Model file for the job. Use its own axes, mm. Face numbers are marked on the shaded views. A direction names the side the tool comes from. Give positions to 0.01 mm unless a question says otherwise; leave off trailing zeros. Loops run counter-clockwise (first coordinate to the right, second up) from the corner with the lowest first, then second, coordinate; pieces in that order, holes last. Notation, with made-up numbers: M 14,18 L 65,18 A24 ccw 65,51 Z; hole C 27.25,85 d7. An arc over 180 degrees is marked long. Use CSV: the item, a comma, the result in double quotes. Start each with the question number.
(1) Two-plate mould, pull along X, no slides. Class the marked faces 1, 2 and 3: pulls with the +X half, pulls with the -X half, needs draft (parallel to the pull), parting line crosses it, or undercut.
(2) Flat gauge pins, fed straight in: P1, Ø1.2, axis at x = -3, y = 15.5, coming from the -Z side; P2, Ø2, axis at x = 1, y = 7.5, coming from the +Z side; P3, Ø3, axis at x = -3, y = 2.5, coming from the -Z side; P4, Ø3, axis at x = 1.5, z = 0.5, coming from the -Y side. Where does each tip first touch, or does it go through?
(3) Wall check: line 1 along X through (y, z) = (14.75, 3.25); line 2 along Z through (x, y) = (1.25, 10.75); line 3 along Y through (x, z) = (0.25, 1.5). Give the ranges that are in metal, low to high. Write a range as from..to.
(4) Slice it at C-C on y = 7. List the corners of the cut face in (x, z).
(5) Tool access for the marked faces 4 and 5: list every direction of +Z, -Z, +X, -X, +Y, -Y with a clear straight run to the whole face (end or side of a thin tool).
(6) Slice it at D-D on y = 14. List the corners of the cut face in (x, z), and give its area (3 significant figures).
(7) Slice it at A-A on x = 0. List the corners of the cut face in (y, z), and give its area (4 significant figures).
(8) Slice it at B-B on z = 0. List the corners of the cut face in (x, y).
```python
from build123d import *

# Parameters (mm, degrees)
SKETCH1_R           = 3
BOSS_EXTRUDE1_DEPTH = 13
CUT_EXTRUDE1_DEPTH  = 1.5
FILLET1_R           = 1
FILLET2_R           = 1
FILLET3_R           = 1
FILLET4_R           = 1


with BuildPart() as part:
    # Sketch1 → Boss-Extrude1 (new body)
    with BuildSketch(Plane(origin=(0, 0, 0), x_dir=(1, 0, 0), z_dir=(0, 1, 0))):
        with Locations(Location((0, 0, 0), (0, 0, 90))):
            Circle(SKETCH1_R)
    extrude(amount=BOSS_EXTRUDE1_DEPTH)

    # Sketch3 → Revolve2 (revolve)
    with BuildSketch(Plane.XY, mode=Mode.PRIVATE) as revolve2_sk:
        Polygon((0, 13), (0, 16), (-5.5, 16), (-3, 13), align=None)
    revolve(revolve2_sk.sketch.rotate(Axis((0, 13, 0), (0, 1, 0)), 270), axis=Axis((0, 13, 0), (0, 1, 0)))

    # Sketch4 → Cut-Extrude1 (cut)
    with BuildSketch(Plane(origin=(0, 16, 0), x_dir=(1, 0, 0), z_dir=(0, 1, 0))):
        Polygon((-0.819580165, 0.819580165), (-3.693115778, 0.819580165), (-3.693115778, -0.819580165), (-0.819580165, -0.819580165), (-0.819580165, -3.693115778), (0.819580165, -3.693115778), (0.819580165, -0.819580165), (3.693115778, -0.819580165), (3.693115778, 0.819580165), (0.819580165, 0.819580165), (0.819580165, 3.693115778), (-0.819580165, 3.693115778), align=None)
    extrude(amount=-CUT_EXTRUDE1_DEPTH, mode=Mode.SUBTRACT)

    # Fillet1
    fillet1_edges = [part.edges().sort_by_distance(p)[0] for p in [
        (0, 14.5, -3.693115778),
    ]]
    fillet(fillet1_edges, radius=FILLET1_R)

    # Fillet2
    fillet2_edges = [part.edges().sort_by_distance(p)[0] for p in [
        (3.693115778, 14.5, 0),
    ]]
    fillet(fillet2_edges, radius=FILLET2_R)

    # Fillet3
    fillet3_edges = [part.edges().sort_by_distance(p)[0] for p in [
        (0, 14.5, 3.693115778),
    ]]
    fillet(fillet3_edges, radius=FILLET3_R)

    # Fillet4
    fillet4_edges = [part.edges().sort_by_distance(p)[0] for p in [
        (-3.693115778, 14.5, 0),
    ]]
    fillet(fillet4_edges, radius=FILLET4_R)


solid = part.part
```
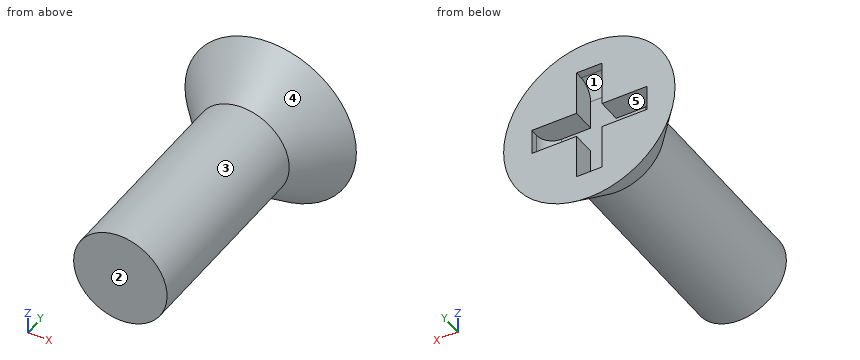
Reply:
1,face 1,"undercut"
1,face 2,"needs draft"
1,face 3,"parting line crosses it"
2,P1,"stops at z = -4.81"
2,P2,"stops at z = 3"
2,P3,"stops at z = -2.6"
2,P4,"stops at y = 0"
3,line 1,"x = -3.05..-0.82, 0.82..3.05"
3,line 2,"z = -2.73..2.73"
3,line 3,"y = 0..14.5"
4,outline,"C 0,0 d6"
5,face 4,"-Y"
5,face 5,"+Y"
6,outline,"C 0,0 d7.67"
6,area,"46.2 mm^2"
7,outline,"M 0,-3 L 13,-3 L 16,-5.5 L 16,-3.69 L 15.5,-3.69 A1 cw 14.5,-2.69 L 14.5,2.69 A1 cw 15.5,3.69 L 16,3.69 L 16,5.5 L 13,3 L 0,3 Z"
7,area,"92.85 mm^2"
8,outline,"M -5.5,16 L -3,13 L -3,0 L 3,0 L 3,13 L 5.5,16 L 3.69,16 L 3.69,15.5 A1 cw 2.69,14.5 L -2.69,14.5 A1 cw -3.69,15.5 L -3.69,16 Z"
